Part model, mm, in its own coordinate system. Face numbers are marked on the shaded views. A direction names the side the tool comes from. Coordinates: 2 decimals unless noted, no trailing zeros. Order: outer loops, then holes, each group sorted by start corner. A loop starts at its lowest first (then second) coordinate and runs counter-clockwise, first axis right, second up. Notation, with made-up numbers: (79, 65.5) - (105, 65.5) arc R22 cw to (105, 91.5) - close; hole circle Ø5 at (-38.5, 66.25). An arc over 180 degrees is marked (long way). Use a Markdown table: item, result. Add a question column.
1) Two-plate mould, pull along Z, no slides. Class the marked faces 1, 2, 3 and 4: +Z half, -Z half, draft (parallel to the pull), parting line (faces both ways), or undercut.
2) Saw through at C-C on z = 12.25. List the corners of the cut face in (x, y).
3) Drop flat-ended pins along their axis: P1, Ø3, axis at x = -15, z = 16, coming from the -Y side; P2, Ø1, axis at y = -5.5, z = 6, coming from the -X side; P3, Ø3, axis at y = -5, z = 13, coming from the +X side; P4, Ø7.5, axis at x = -16, z = 11, coming from the +Y side. Give the stop position or say it passes through.
4) Saw through at D-D on y = -9.25. List the corners of the cut face in (x, z), then the cut area to 3 significant figures.
5) Saw through at B-B on y = -5.25. List the corners of the cut face in (x, z).
6) Tool access for the marked faces 5, 6, 7 and 8: list every direction of +Z, -Z, +X, -X, +Y, -Y with a clear straight run to the whole face (end or side of a thin tool).
7) Saw through at A-A on x = -15. List the corners of the cut face in (y, z).
8) Wall check: L1, parallel to X at y = -8.85, z = 16; L2, parallel to Z at x = -15, y = -8.5; L3, parallel to Y at x = 12, z = 12.5. Give the ranges that are in metal, low to high. Write a range as [from, to].
```python
from build123d import *

# Parameters (mm, degrees)
F1_DEPTH = 20
F2_DEPTH = 2
F4_DEPTH = 25


with BuildPart() as f1:
    # F0 (on Top) → F1 (new body)
    with BuildSketch(Plane.XY):
        with BuildLine():
            ThreePointArc((-6.689544, -7.7), (-8.302401, -5.92538), (-9.456362, -3.823248))
            Line((-9.456362, -3.823248), (-11.689544, -3.823248))
            Line((-11.689544, -3.823248), (-11.689544, -7.323248))
            Line((-11.689544, -7.323248), (-18.689544, -7.323248))
            Line((-18.689544, -7.323248), (-18.689544, -10.823248))
            Line((-18.689544, -10.823248), (18.689544, -10.823248))
            Line((18.689544, -10.823248), (18.689544, -7.323248))
            Line((18.689544, -7.323248), (11.689544, -7.323248))
            Line((11.689544, -7.323248), (11.689544, -3.823248))
            Line((11.689544, -3.823248), (9.456362, -3.823248))
            ThreePointArc((9.456362, -3.823248), (8.302401, -5.92538), (6.689544, -7.7))
            Line((6.689544, -7.7), (-6.689544, -7.7))
        make_face()
    extrude(amount=F1_DEPTH)

    # F0 (on Top) → F2 (join)
    with BuildSketch(Plane.XY):
        with BuildLine():
            ThreePointArc((-6.689544, -7.7), (-8.302401, -5.92538), (-9.456362, -3.823248))
            Line((-9.456362, -3.823248), (-11.689544, -3.823248))
            Line((-11.689544, -3.823248), (-11.689544, -7.323248))
            Line((-11.689544, -7.323248), (-18.689544, -7.323248))
            Line((-18.689544, -7.323248), (-18.689544, -10.823248))
            Line((-18.689544, -10.823248), (18.689544, -10.823248))
            Line((18.689544, -10.823248), (18.689544, -7.323248))
            Line((18.689544, -7.323248), (11.689544, -7.323248))
            Line((11.689544, -7.323248), (11.689544, -3.823248))
            Line((11.689544, -3.823248), (9.456362, -3.823248))
            ThreePointArc((9.456362, -3.823248), (8.302401, -5.92538), (6.689544, -7.7))
            Line((6.689544, -7.7), (-6.689544, -7.7))
        make_face()
    extrude(amount=F2_DEPTH)

    # F3 (on face) → F4 (cut)
    with BuildSketch(Plane(origin=(0, -7.323248, 0), x_dir=(-1, 0, 0), z_dir=(0, 1, 0))):
        with BuildLine():
            Line((-13.25, 16), (-15, 16))
            Line((-15, 16), (-15, 14.25))
            ThreePointArc((-15, 14.25), (-13.762563, 14.762563), (-13.25, 16))
        make_face()
        with BuildLine():
            Line((-15, 14.25), (-15, 16))
            Line((-15, 16), (-13.25, 16))
            ThreePointArc((-13.25, 16), (-16.237437, 17.237437), (-15, 14.25))
        make_face()
        with BuildLine():
            ThreePointArc((16.75, 4), (15, 5.75), (13.25, 4))
            ThreePointArc((13.25, 4), (15, 2.25), (16.75, 4))
        make_face()
        with BuildLine():
            ThreePointArc((-13.25, 4), (-13.762563, 5.237437), (-15, 5.75))
            Line((-15, 5.75), (-15, 4))
            Line((-15, 4), (-13.25, 4))
        make_face()
        with BuildLine():
            Line((-15, 4), (-15, 5.75))
            ThreePointArc((-15, 5.75), (-16.237437, 2.762563), (-13.25, 4))
            Line((-13.25, 4), (-15, 4))
        make_face()
        with BuildLine():
            ThreePointArc((16.75, 16), (15, 17.75), (13.25, 16))
            ThreePointArc((13.25, 16), (15, 14.25), (16.75, 16))
        make_face()
    extrude(amount=-F4_DEPTH, mode=Mode.SUBTRACT)


solid = f1.part
```
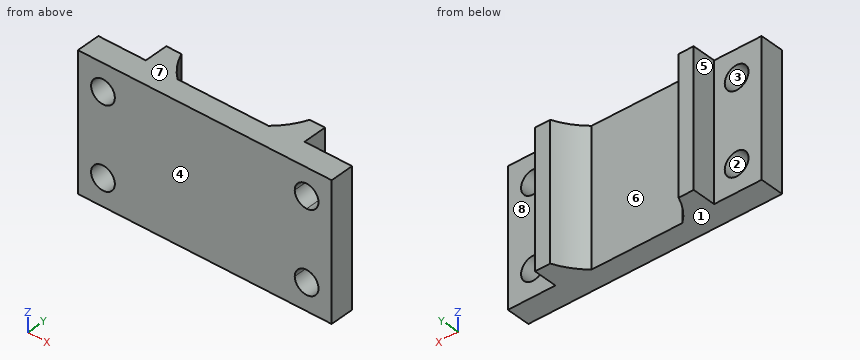
Results are:
| question | item | result |
|---|---|---|
| 1 | face 1 | -Z half |
| 1 | face 2 | undercut |
| 1 | face 3 | undercut |
| 1 | face 4 | draft |
| 2 | outline | (-18.69, -10.82) - (18.69, -10.82) - (18.69, -7.32) - (11.69, -7.32) - (11.69, -3.82) - (9.46, -3.82) arc R10.2 cw to (6.69, -7.7) - (-6.69, -7.7) arc R10.2 cw to (-9.46, -3.82) - (-11.69, -3.82) - (-11.69, -7.32) - (-18.69, -7.32) - close |
| 3 | P1 | through |
| 3 | P2 | x = -11.69 |
| 3 | P3 | x = 11.69 |
| 3 | P4 | y = -7.32 |
| 4 | outline | (-18.69, 0) - (18.69, 0) - (18.69, 20) - (-18.69, 20) - close; hole circle Ø3.5 at (-15, 4); hole circle Ø3.5 at (-15, 16); hole circle Ø3.5 at (15, 4); hole circle Ø3.5 at (15, 16) |
| 4 | area | 709 mm2 |
| 5 | outline | (-11.69, 0) - (-8.75, 0) - (-8.75, 20) - (-11.69, 20) - close; (8.75, 0) - (11.69, 0) - (11.69, 20) - (8.75, 20) - close |
| 6 | face 5 | +Z, -Z, -X, +Y |
| 6 | face 6 | +Z, -Z, +Y |
| 6 | face 7 | +Z, +X, -X, +Y, -Y |
| 6 | face 8 | +Z, -Z, +X, +Y |
| 7 | outline | (-10.82, 0) - (-7.32, 0) - (-7.32, 2.25) - (-10.82, 2.25) - close; (-10.82, 5.75) - (-7.32, 5.75) - (-7.32, 14.25) - (-10.82, 14.25) - close; (-10.82, 17.75) - (-7.32, 17.75) - (-7.32, 20) - (-10.82, 20) - close |
| 8 | L1 | [-18.69, -16.75], [-13.25, 13.25], [16.75, 18.69] |
| 8 | L2 | [0, 2.25], [5.75, 14.25], [17.75, 20] |
| 8 | L3 | [-10.82, -7.32] |
